Design review of the part built by this model. Coordinates are the model's own, in mm. A direction names the side the tool comes from. Round coordinates to 2 decimals unless told otherwise and drop trailing zeros. Write each loop counter-clockwise with the first axis right and the second up, starting at its lowest first coordinate (ties: lowest second). Pieces come first, ordered by that corner, then holes. Notation, with made-up numbers: M 15,69 L 48,69 A25 ccw 48,87 Z; hole C -15.75,37.5 d4. An arc over 180 degrees is marked long. Use CSV: the item, a comma, the result in double quotes.
from build123d import *

# Parameters (mm, degrees)
SKETCH1_W          = 19.05
SKETCH1_H          = 2.0828
CHAMFER1_SIZE      = 0.5953125
SKETCH4_R          = 3.9624
EXTRUDE1_DEPTH     = 2.2098
CUT_EXTRUDE1_DEPTH = 1.1049


with BuildPart() as part:
    # Sketch1 → Revolve1 (revolve)
    with BuildSketch(Plane(origin=(0, 0, 0), x_dir=(0, 0, -1), z_dir=(1, 0, 0))):
        with Locations((9.525, 1.0414)):
            Rectangle(SKETCH1_W, SKETCH1_H)
    revolve(axis=Axis((0, 0, 0), (0, 0, 1)))

    # Chamfer1
    chamfer1_edges = [part.edges().sort_by_distance(p)[0] for p in [
        (0, -2.0828, -19.05),
    ]]
    chamfer(chamfer1_edges, length=CHAMFER1_SIZE)

    # Sketch4 → Extrude1 (add)
    with BuildSketch(Plane.XY):
        Circle(SKETCH4_R)
    extrude(amount=EXTRUDE1_DEPTH)

    # Sketch9 → Cut-Revolve3 (revolve, cut)
    with BuildSketch(Plane(origin=(0, 0, 0), x_dir=(0, 0, -1), z_dir=(1, 0, 0))):
        with BuildLine():
            Line((0, 3.9624), (-0.381, 3.9624))
            ThreePointArc((-0.381, 3.9624), (-1.434442989, 3.157885071), (-2.2098, 2.0828))
            Line((-2.2098, 2.0828), (-2.5908, 2.0828))
            Line((-2.5908, 2.0828), (-2.5908, 4.3434))
            Line((-2.5908, 4.3434), (0, 4.3434))
            Line((0, 4.3434), (0, 3.9624))
        make_face()
    revolve(axis=Axis((0, 0, 0), (0, 0, 1)), mode=Mode.SUBTRACT)

    # Sketch6 → Cut-Extrude1 (cut)
    with BuildSketch(Plane.XY.offset(2.2098)):
        Polygon((0, -1.374815329), (1.190625, -0.687407664), (1.190625, 0.687407664), (0, 1.374815329), (-1.190625, 0.687407664), (-1.190625, -0.687407664), align=None)
    extrude(amount=-CUT_EXTRUDE1_DEPTH, mode=Mode.SUBTRACT)


solid = part.part
1) Add section A-A on y = 0. Write out the cut boundary in (x, z), then the cut area to 3 significant figures.
Answers:
outline,"M -3.96,0 L -2.08,0 L -2.08,-18.45 L -1.49,-19.05 L 1.49,-19.05 L 2.08,-18.45 L 2.08,0 L 3.96,0 L 3.96,0.38 A4.53 ccw 2.08,2.21 L 1.19,2.21 L 1.19,1.1 L -1.19,1.1 L -1.19,2.21 L -2.08,2.21 A4.53 ccw -3.96,0.38 Z"
area,"91.1 mm²"
2) The part is to be moulded in two halves that separate along X. For faces 3 (the face through (2, -2, 0)), 4 (the face through (0.587, -1.036, 1.665)), 5 (the face through (-0.626, 1.987, -9.357)), say which applies: released by +X, released by -X, zero draft, split by the parting line, or undercut.
Answers:
face 3,"zero draft"
face 4,"undercut"
face 5,"split by the parting line"
3) Machinability: for faces 1 (the face through (0.6, 1.03, 1.67)), 2 (the face through (3.66, -1.52, 0.19)), which of the approach directions +Z, -Z, +X, -X, +Y, -Y give a long, thin tool a straight path to every point of the face, cutting with its end or side? Answer none if there is none.
Answers:
face 1,"+Z"
face 2,"+Z, -Z"
4) For pin 1 Ø1.5 at (y, z) = (3, -13) entering from -X; pin 2 Ø0.6 at (y, z) = (0, 2) entering from +X, all flat-tipped, find the tip position at first contact; note any pin that passes through.
Answers:
pin 1,"through"
pin 2,"x = 2.86"
5) Add section B-B on z = -16.75. Write out the cut boundary in (x, y), then the cut area to 3 significant figures.
Answers:
outline,"C 0,0 d4.17"
area,"13.6 mm²"
6) Wall thickness on line 1 along Z through (x, y) = (-1, -0.75); line 2 along X through (y, z) = (-1.75, -7.5): over which ranges is each line inside the solid? List them lowest first. Write a range as [from, to].
Answers:
line 1,"[-19.05, 1.1]"
line 2,"[-1.13, 1.13]"
